from build123d import *

# Parameters (mm, degrees)
SKETCH_1_W          = 40
SKETCH_1_H          = 40
EXTRUDE_1_DEPTH     = 20
SKETCH_2_R          = 6.25
EXTRUDE_2_DEPTH     = 1.5
SKETCH_3_R          = 3
EXTRUDE_776_DEPTH   = 4.5
EXTRUDE_START       = 1.5
SKETCH_4_R          = 6.25
EXTRUDE_4_DEPTH     = 1.5
EXTRUDE_START_2     = 3.7
SKETCH_5_R          = 3
EXTRUDE_5_DEPTH     = 3.7
SKETCH_7_R          = 0.75
CUT_EXTRUDE_1_DEPTH = 5
SKETCH_8_R          = 0.75
CUT_EXTRUDE_2_DEPTH = 5
EXTRUDE_6_DEPTH     = 1
EXTRUDE_1947_DEPTH  = 4
EXTRUDE_1947_TAPER  = 6
CUT_EXTRUDE_3_DEPTH = 65.156059729
FILLET_1_R          = 2


with BuildPart() as part:
    # Эскиз1 → Бобышка-Вытянуть1 (new body)
    with BuildSketch(Plane(origin=(0, 0, 0), x_dir=(1, 0, 0), z_dir=(0, 1, 0))):
        with Locations((20, -20)):
            Rectangle(SKETCH_1_W, SKETCH_1_H)
    extrude(amount=EXTRUDE_1_DEPTH)

    # Эскиз2 → Бобышка-Вытянуть2 (add)
    with BuildSketch(Plane.XY.offset(40)):
        with Locations(Location((30, 10, 0), (0, 0, 180))):
            Circle(SKETCH_2_R)
    extrude(amount=EXTRUDE_2_DEPTH)

    # Эскиз3 → Extrude 776 (add)
    with BuildSketch(Plane.XY.offset(41.5)):
        with Locations((30, 10)):
            Circle(SKETCH_3_R)
    extrude(amount=EXTRUDE_776_DEPTH)

    # Эскиз4 → Бобышка-Вытянуть4 (add)
    with BuildSketch(Plane(origin=(0, 0, 0), x_dir=(-1, 0, 0), z_dir=(0, 0, -1)).offset(EXTRUDE_START)):
        with Locations((-30, 10)):
            Circle(SKETCH_4_R)
    extrude(amount=-EXTRUDE_4_DEPTH)

    # Эскиз5 → Бобышка-Вытянуть5 (add)
    with BuildSketch(Plane(origin=(0, 0, -1.5), x_dir=(-1, 0, 0), z_dir=(0, 0, -1)).offset(EXTRUDE_START_2)):
        with Locations(Location((-30, 10, 0), (0, 0, 180))):
            Circle(SKETCH_5_R)
    extrude(amount=-EXTRUDE_5_DEPTH)

    # Эскиз7 → Вырез-Вытянуть1 (cut)
    with BuildSketch(Plane(origin=(0, 0, 0), x_dir=(-1, 0, 0), z_dir=(0, 0, -1))):
        with Locations((-17.5, 17.5)):
            Circle(SKETCH_7_R)
        with Locations((-2.5, 17.5)):
            Circle(SKETCH_7_R)
        with Locations((-2.5, 2.5)):
            Circle(SKETCH_7_R)
        with Locations((-17.5, 2.5)):
            Circle(SKETCH_7_R)
    extrude(amount=-CUT_EXTRUDE_1_DEPTH, mode=Mode.SUBTRACT)

    # Эскиз8 → Вырез-Вытянуть2 (cut)
    with BuildSketch(Plane.XY.offset(40)):
        with Locations((10, 17)):
            Circle(SKETCH_8_R)
        with Locations((3, 10)):
            Circle(SKETCH_8_R)
        with Locations((10, 3)):
            Circle(SKETCH_8_R)
    extrude(amount=-CUT_EXTRUDE_2_DEPTH, mode=Mode.SUBTRACT)

    # Эскиз9 → Бобышка-Вытянуть6 (add)
    with BuildSketch(Plane(origin=(40, 0, 0), x_dir=(0, 0, -1), z_dir=(1, 0, 0))):
        Polygon((-6.5, 10), (-6.5, 13.5), (-10.5, 13.5), (-10.5, 6.5), (-6.5, 6.5), align=None)
    extrude(amount=EXTRUDE_6_DEPTH)

    # Эскиз10 → Extrude 1947 (add)
    with BuildSketch(Plane(origin=(41, 0, 0), x_dir=(0, 0, -1), z_dir=(1, 0, 0))):
        Polygon((-7.5, 12.5), (-8.5, 12.5), (-9.5, 12.5), (-9.5, 7.5), (-7.5, 7.5), align=None)
    extrude(amount=EXTRUDE_1947_DEPTH, taper=EXTRUDE_1947_TAPER)

    # Эскиз11 → Вырез-Вытянуть3 (cut, through all)
    with BuildSketch(Plane(origin=(40, 0, 0), x_dir=(0, 0, -1), z_dir=(1, 0, 0))):
        Polygon((-40, 20), (-38, 20), (-40, 19), align=None)
        Polygon((0, 20), (-2, 20), (0, 19), align=None)
        Polygon((0, 0), (-2, 0), (0, 1), align=None)
        Polygon((-40, 0), (-38, 0), (-40, 1), align=None)
    extrude(amount=-CUT_EXTRUDE_3_DEPTH, mode=Mode.SUBTRACT)

    # Скругление1
    fillet_1_edges = [part.edges().sort_by_distance(p)[0] for p in [
        (0, 0, 20),
        (0, 20, 20),
        (40, 0, 20),
        (40, 20, 20),
    ]]
    fillet(fillet_1_edges, radius=FILLET_1_R)


solid = part.part
The listing builds one solid part. Answer for the finished solid, in the listing's coordinates (mm). A direction names the side the tool comes from. Give positions to 0.01 mm unless a question says otherwise; leave off trailing zeros. Write each loop counter-clockwise with the first axis right and the second up, starting at its lowest first coordinate (ties: lowest second). Pieces come first, ordered by that corner, then holes.
Item 1: Determine the mould class of faces 1 (the cylindrical face through (39.4, 19.43, 19.72)), 2 (the cylindrical face through (18.095, 2.044, 2.465)), 3 (the flat face through (30, 10, -5.2)) for opening direction Y: released by +Y, released by -Y, zero draft, split by the parting line, or undercut.
Item 2: Section D-D, the plane x = 15.5 is taken. Write down the section's boundary in (y, z), plus the area to 3 significant figures.
Item 3: Which of the six approach directions +Z, -Z, +X, -X, +Y, -Y give full straight-line access (tool end or side, diameter ignored) to faces 4 (the flat face through (2.5, 2.5, 5)), 5 (the flat face through (20, 0, 20)), 6 (the flat face through (10, 17, 35))?
Item 4: Section B-B, the plane z = 27 is taken. Write down the section's boundary in (x, y).
Item 5: Section C-C, the plane x = 30 is taken. Write down the section's boundary in (y, z).
Item 6: Find the intervals of material crossed by line 1 along Y through (x, z) = (10, 37.1); line 2 along Y through (x, z) = (2, 4); line 3 along Z through (x, y) = (39.5, 18), in increasing order.
Item 7: Flat-ended cylindrical pins translate along their axes: P1, Ø3, axis at y = 18, z = 23, coming from the +X side; P2, Ø8, axis at x = 36.5, y = 2.5, coming from the +Z side; P3, Ø0.8, axis at x = 9.5, y = 17, coming from the +Z side. Find the tip coordinate at first contact, or state that the pin passes through.
Item 8: Section A-A, the plane x = 10 is taken. Write down the section's boundary in (y, z).
Completed:
1. face 1: released by +Y
1. face 2: undercut
1. face 3: zero draft
2. outline: (0, 2) - (1, 0) - (19, 0) - (20, 2) - (20, 38) - (19, 40) - (1, 40) - (0, 38) - close
2. area: 796 mm2
3. face 4: -Z
3. face 5: +Z, -Z, +X, -X, -Y
3. face 6: +Z
4. outline: (0, 2) arc R2 ccw to (2, 0) - (38, 0) arc R2 ccw to (40, 2) - (40, 18) arc R2 ccw to (38, 20) - (2, 20) arc R2 ccw to (0, 18) - close
5. outline: (0, 2) - (1, 0) - (3.75, 0) - (3.75, -1.5) - (7, -1.5) - (7, -5.2) - (13, -5.2) - (13, -1.5) - (16.25, -1.5) - (16.25, 0) - (19, 0) - (20, 2) - (20, 38) - (19, 40) - (16.25, 40) - (16.25, 41.5) - (13, 41.5) - (13, 46) - (7, 46) - (7, 41.5) - (3.75, 41.5) - (3.75, 40) - (1, 40) - (0, 38) - close
6. line 1: y = 0 to 2.25, 3.75 to 16.25, 17.75 to 20
6. line 2: y = 0 to 1.94, 3.06 to 16.94, 18.06 to 20
6. line 3: z = 0 to 40
7. P1: stops at x = 40
7. P2: stops at z = 41.5
7. P3: stops at z = 40
8. outline: (0, 2) - (1, 0) - (19, 0) - (20, 2) - (20, 38) - (19, 40) - (17.75, 40) - (17.75, 35) - (16.25, 35) - (16.25, 40) - (3.75, 40) - (3.75, 35) - (2.25, 35) - (2.25, 40) - (1, 40) - (0, 38) - close
